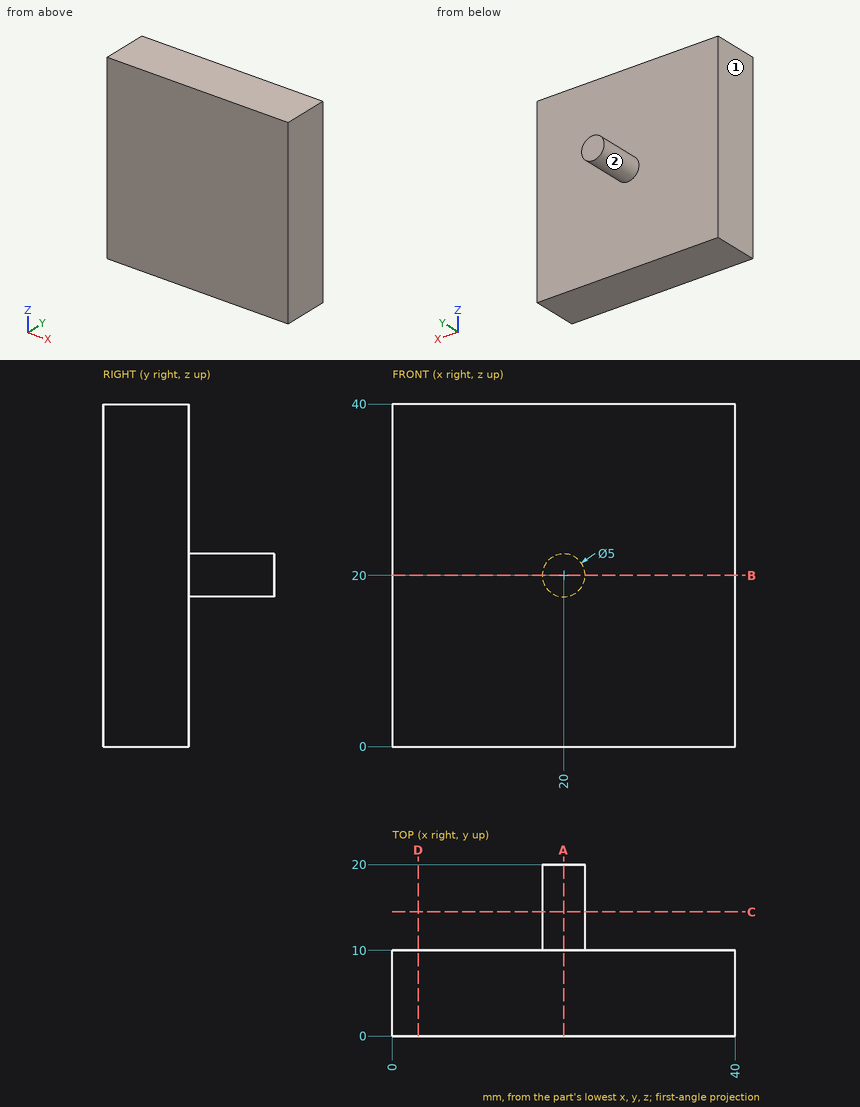
For this review, use the dimensioned drawing (mm, ordinates from the lowest corner) and the shaded views. A direction names the side the tool comes from. Round coordinates to 2 decimals unless told otherwise and drop trailing zeros. Write each loop counter-clockwise with the first axis right and the second up, starting at its lowest first coordinate (ties: lowest second). Pieces come first, ordered by that corner, then holes. Notation, with made-up numbers: (-30.5, 45) -> (-13.5, 45) arc R3 cw to (-13.5, 49) -> close; hole circle Ø8 at (-11, 30). An arc over 180 degrees is marked (long way). Use CSV: the item, a comma, the result in double quotes.
(1) Consider section B-B, the plane z = 20. Give the boundary of the cut face in (x, y), plus the area to 3 significant figures.
Computed values:
outline,"(0, 0) -> (40, 0) -> (40, 10) -> (22.5, 10) -> (22.5, 20) -> (17.5, 20) -> (17.5, 10) -> (0, 10) -> close"
area,"450 mm²"
(2) Consider section C-C, the plane y = 14.5. Give the boundary of the cut face in (x, z).
Computed values:
outline,"circle Ø5 at (20, 20)"
(3) For the marked faces 1 and 2, list the 3-axis set-ups (+Z, -Z, +X, -X, +Y, -Y) from which the entire face can be reached by the end or side of a thin tool; tool diameter is ignored.
Computed values:
face 1,"+Z, -Z, -X, +Y, -Y"
face 2,"+Y"
(4) Consider section D-D, the plane x = 3. Give the boundary of the cut face in (y, z).
Computed values:
outline,"(0, 0) -> (10, 0) -> (10, 40) -> (0, 40) -> close"
(5) Clearance check with flat-ended pins moving along their axes: P1, Ø6, axis at x = 14, z = 9.5, coming from the +Y side; P2, Ø1.5, axis at x = 26.5, y = 11, coming from the +Z side; P3, Ø4, axis at x = 21.5, y = 13, coming from the -Z side. State where each tip first meets the part, or that it passes through.
Computed values:
P1,"y = 10"
P2,"through"
P3,"z = 17.5"
(6) Consider section A-A, the plane x = 20. Give the boundary of the cut face in (y, z).
Computed values:
outline,"(0, 0) -> (10, 0) -> (10, 17.5) -> (20, 17.5) -> (20, 22.5) -> (10, 22.5) -> (10, 40) -> (0, 40) -> close"
(7) To check wall thickness, follow L1, parallel to Y at x = 26.5, z = 22; L2, parallel to Z at x = 22, y = 18. State the ranges of each line that lie inside material, in increasing order. Write a range as [from, to].
Computed values:
L1,"[0, 10]"
L2,"[18.5, 21.5]"
